from build123d import *

# Parameters (mm, degrees)
F0_R     = 38.1
F1_DEPTH = 76.2
F2_R     = 35.56
F3_DEPTH = 71.12
F4_SIZE  = 5.08


with BuildPart() as f1:
    # F0 (on Top) → F1 (new body)
    with BuildSketch(Plane.XY):
        Circle(F0_R)
    extrude(amount=F1_DEPTH)

    # F2 (on face) → F3 (cut)
    with BuildSketch(Plane.XY.offset(76.2)):
        Circle(F2_R)
    extrude(amount=-F3_DEPTH, mode=Mode.SUBTRACT)

    # F4
    f4_edges = [f1.edges().sort_by_distance(p)[0] for p in [
        (-38.1, 0, 0),
    ]]
    chamfer(f4_edges, length=F4_SIZE)


solid = f1.part
Source: CAD feature listing. Evaluate the final solid. Frame: model axes, mm. A direction names the side the tool comes from. Round coordinates to 2 decimals unless told otherwise and drop trailing zeros. Write each loop counter-clockwise with the first axis right and the second up, starting at its lowest first coordinate (ties: lowest second). Pieces come first, ordered by that corner, then holes. Notation, with made-up numbers: (67.25, 70) - (86.25, 70) arc R15 ccw to (86.25, 74) - close; hole circle Ø11 at (18.5, -32). An arc over 180 degrees is marked (long way). Use CSV: the item, a comma, the result in double quotes. Start each with the question number.
(1) Cut plane C-C, the plane z = 15. Return loops of the section in (x, y).
(2) Set-up query: faces 1 (the face through (0, 0, 5.08)), 2 (the face through (34, 11, 76.2)). Return all of +Z, -Z, +X, -X, +Y, -Y with unobstructed straight access to the full face (end or side cutting, diameter ignored); none if empty.
(3) Mould query, pull axis X, two halves, no side actions, for faces 3 (the face through (0, 0, 0)), 4 (the face through (-7.709, -34.714, 41.138)), 5 (the face through (-30.235, -23.183, 40.142)). Classes: pulls with the +X half, pulls with the -X half, needs draft (parallel to the pull), parting line crosses it, or undercut.
(4) First-contact query: pin 1 Ø3 at (y, z) = (-7, 19) entering from -X; pin 2 Ø21.5 at (x, y) = (3, -16.5) entering from +Z; pin 3 Ø8 at (y, z) = (22.5, 9.5) entering from +X. Flat tips, straight axial feed; report the tip coordinate or a pass-through.
(5) Material intervals for probe 1 along Y at (x, z) = (-1, 46.5); probe 2 along Z at (x, y) = (-7.5, 21); probe 3 along Y at (x, z) = (18.5, 48), sorted ascending. Write a range as [from, to].
(6) Cut plane A-A, the plane x = 0. Return loops of the section in (y, z), and give its area (3 significant figures).
Geometry says:
1,outline,"circle Ø76.2 at (0, 0); hole circle Ø71.12 at (0, 0)"
2,face 1,"+Z"
2,face 2,"+Z, +X, -X, +Y, -Y"
3,face 3,"needs draft"
3,face 4,"undercut"
3,face 5,"parting line crosses it"
4,pin 1,"x = -37.7"
4,pin 2,"z = 5.08"
4,pin 3,"x = 33.31"
5,probe 1,"[-38.09, -35.55], [35.55, 38.09]"
5,probe 2,"[0, 5.08]"
5,probe 3,"[-33.31, -30.37], [30.37, 33.31]"
6,outline,"(-38.1, 5.08) - (-33.02, 0) - (33.02, 0) - (38.1, 5.08) - (38.1, 76.2) - (35.56, 76.2) - (35.56, 5.08) - (-35.56, 5.08) - (-35.56, 76.2) - (-38.1, 76.2) - close"
6,area,"723 mm²"
